```python
from build123d import *

# Parameters (mm, degrees)
F0_R     = 1.75
F1_DEPTH = 15
F2_R     = 2.5
F2_R_2   = 1.75
F3_DEPTH = 0.6


# Not quite as in the source:
# - a pattern or mirror of a feature is missing from the dataset's text; its kind, count and spacing are read off the source's solid


with BuildPart() as f1:
    # F0 (on Front) → F1 (new body, symmetric)
    with BuildSketch(Plane.XZ):
        Circle(F0_R)
    extrude(amount=F1_DEPTH, both=True)

    # F2 (on face) → F3 (join)
    with BuildSketch(Plane.XZ.offset(15)):
        Circle(F2_R)
        Circle(F2_R_2, mode=Mode.SUBTRACT)
        Circle(F2_R_2)
    f3 = extrude(amount=F3_DEPTH)

    # F3_copies: F3 across plane
    add(f3.mirror(Plane.ZX))

    # F4 (on Top) → F5 (revolve)
    with BuildSketch(Plane.XY):
        with BuildLine():
            Line((0, -16.9), (0, -15.6))
            Line((0, -15.6), (-2.5, -15.6))
            ThreePointArc((-2.5, -15.6), (-1.4089002804, -16.5555774622), (0, -16.9))
        make_face()
    f5 = revolve(axis=Axis((0, -16.1810277431, 0), (0, -1, 0)))

    # F5_copies: F5 across plane
    add(f5.mirror(Plane.ZX))


solid = f1.part
```
The model under review builds one solid part; all positions refer to its coordinate system, in mm. A direction names the side the tool comes from. Give positions to 0.01 mm unless a question says otherwise; leave off trailing zeros. Order: outer loops, then holes, each group sorted by start corner. A loop starts at its lowest first (then second) coordinate and runs counter-clockwise, first axis right, second up. Notation, with made-up numbers: (89, 10) - (129, 10) arc R25 cw to (129, 31) - close; hole circle Ø8 at (64.5, 47.5). An arc over 180 degrees is marked (long way). Use CSV: the item, a comma, the result in double quotes. Start each with the question number.
Q1. We need section D-D, the plane y = 7. Write out the cut boundary in (x, z).
Q2. Clearance check with flat-ended pins moving along their axes: pin 1 Ø1.5 at (x, z) = (-0.5, 0) entering from -Y; pin 2 Ø1.5 at (x, z) = (1, -1) entering from +Y. State where each tip first meets the part, or that it passes through.
Q3. To check wall thickness, follow line 1 along Y through (x, z) = (-1.3, 1.95); line 2 along Y through (x, z) = (1.85, 1.25); line 3 along X through (y, z) = (-13.5, 1.4). State the ranges of each line that lie inside material, in increasing order. Write a range as [from, to].
Q4. Tool access review of faces 1 (the cylindrical face through (-0.54, 15.3, -2.44)), 2 (the flat face through (-2, -15, -1)): name each direction out of +Z, -Z, +X, -X, +Y, -Y from which nothing blocks a thin tool from reaching the whole face with its end or side.
Q5. We need section B-B, the plane z = -2.1. Write out the cut boundary in (x, y), and give its area (3 significant figures).
Q6. We need section A-A, the plane x = 0. Write out the cut boundary in (y, z).
Q7. We need section C-C, the plane z = 0. Write out the cut boundary in (x, y), and give its area (3 significant figures).
Q8. The part is to be moulded in two halves that separate along Y. For faces 3 (the cylindrical face through (1.617, -0.21, -0.67)), 4 (the cylindrical face through (-0.54, -15.3, -2.44)), say which applies: +Y half, -Y half, draft (parallel to the pull), parting line (faces both ways), or undercut.
Outcome:
1,outline,"circle Ø3.5 at (0, 0)"
2,pin 1,"stops at y = -16.9"
2,pin 2,"stops at y = 16.83"
3,line 1,"y = [-15.8, -15], [15, 15.8]"
3,line 2,"y = [-15.93, -15], [15, 15.93]"
3,line 3,"x = [-1.05, 1.05]"
4,face 1,"+Y, -Y"
4,face 2,"none"
5,outline,"(-1.36, -15.6) arc R2.22 ccw to (1.36, -15.6) - (1.36, -15) - (-1.36, -15) - close; (-1.36, 15) - (1.36, 15) - (1.36, 15.6) arc R2.22 ccw to (-1.36, 15.6) - close"
5,area,"4.97 mm^2"
6,outline,"(-15.6, -2.5) - (-15, -2.5) - (-15, -1.75) - (15, -1.75) - (15, -2.5) - (15.6, -2.5) arc R3.05 ccw to (15.6, 2.5) - (15, 2.5) - (15, 1.75) - (-15, 1.75) - (-15, 2.5) - (-15.6, 2.5) arc R3.05 ccw to start"
7,outline,"(-2.5, -15.6) arc R3.05 ccw to (2.5, -15.6) - (2.5, -15) - (1.75, -15) - (1.75, 15) - (2.5, 15) - (2.5, 15.6) arc R3.05 ccw to (-2.5, 15.6) - (-2.5, 15) - (-1.75, 15) - (-1.75, -15) - (-2.5, -15) - close"
7,area,"120 mm^2"
8,face 3,"undercut"
8,face 4,"draft"
